Read the model definition and answer for the solid it produces. Units are mm, in the model's axes. Round coordinates to 2 decimals unless told otherwise and drop trailing zeros. Order: outer loops, then holes, each group sorted by start corner. A loop starts at its lowest first (then second) coordinate and runs counter-clockwise, first axis right, second up.
from build123d import *

# Parameters (mm, degrees)
SCHIZZO1_R                   = 1.5
ESTRUSIONE_ESTRUSIONE1_DEPTH = 3


with BuildPart() as part:
    # Schizzo1 → Estrusione-Estrusione1 (new body)
    with BuildSketch(Plane.XY):
        with BuildLine():
            Line((22, 5), (0, 5))
            ThreePointArc((0, 5), (-5, 0), (0, -5))
            Line((0, -5), (22, -5))
            ThreePointArc((22, -5), (25.445859834, -3.622989098), (26.993725045, -0.250420003))
            Line((26.993725045, -0.250420003), (45.041832618, 3.254653548))
            Line((45.041832618, 3.254653548), (50.666477461, 1.165785339))
            ThreePointArc((50.666477461, 1.165785339), (51.293977461, 1.08172232), (51.921477461, 1.165785339))
            ThreePointArc((51.921477461, 1.165785339), (52.551477461, 1.081007878), (53.181477461, 1.165785339))
            ThreePointArc((53.181477461, 1.165785339), (53.811477461, 1.081063133), (54.441477461, 1.165785339))
            ThreePointArc((54.441477461, 1.165785339), (55.071477461, 1.081063133), (55.701477461, 1.165785339))
            Line((55.701477461, 1.165785339), (55.766477461, 1.165785339))
            ThreePointArc((55.766477461, 1.165785339), (60.745551277, 6.622757917), (54.856357382, 11.082255764))
            Line((54.856357382, 11.082255764), (22, 5))
        make_face()
        Circle(SCHIZZO1_R, mode=Mode.SUBTRACT)
        with Locations((22, 0)):
            Circle(SCHIZZO1_R, mode=Mode.SUBTRACT)
        with Locations((55.766477461, 6.165785339)):
            Circle(SCHIZZO1_R, mode=Mode.SUBTRACT)
    extrude(amount=ESTRUSIONE_ESTRUSIONE1_DEPTH)


solid = part.part
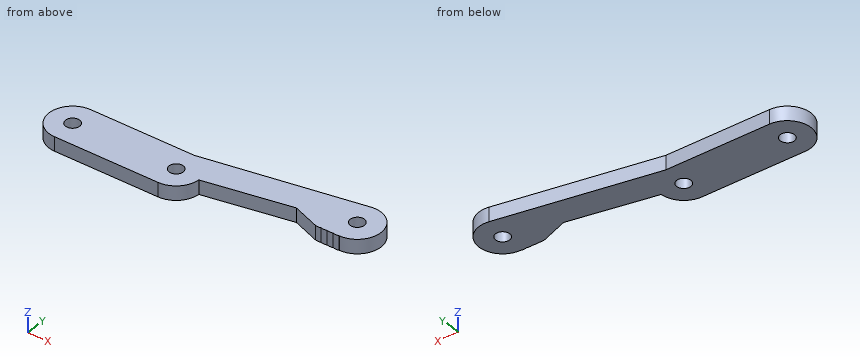
Q1. A cutting plane is placed at A-A, the plane z = 1.5. Give the vertices of the cut face in (x, y), plus the area to 3 significant figures.
Outcome:
outline: (0, -5) - (22, -5) arc R5 ccw to (26.99, -0.25) - (45.04, 3.25) - (50.67, 1.17) arc R2.38 ccw to (51.92, 1.17) arc R2.38 ccw to (53.18, 1.17) arc R2.38 ccw to (54.44, 1.17) arc R2.38 ccw to (55.7, 1.17) - (55.77, 1.17) arc R5 ccw (long way) to (54.86, 11.08) - (22, 5) - (0, 5) arc R5 ccw to start; hole circle Ø3 at (0, 0); hole circle Ø3 at (22, 0); hole circle Ø3 at (55.77, 6.17)
area: 526 mm2
Q2. A cutting plane is placed at B-B, the plane x = 18. Give the vertices of the cut face in (y, z).
Outcome:
outline: (-5, 0) - (5, 0) - (5, 3) - (-5, 3) - close
Q3. Flat-ended cylindrical pins translate along their axes: pin 1 (2.5 mm diameter, centred on x = 0, y = 0, fed in from +Z); pin 2 (1 mm diameter, centred on x = 30.5, z = 2, fed in from +Y); pin 3 (1 mm diameter, centred on x = 10.5, z = 1.5, fed in from +Y). Find the tip coordinate at first contact, or state that the pin passes through.
Outcome:
pin 1: passes through
pin 2: stops at y = 6.67
pin 3: stops at y = 5
Q4. A cutting plane is placed at C-C, the plane y = -3. Give the vertices of the cut face in (x, z), plus the area to 3 significant figures.
Outcome:
outline: (-4, 0) - (26, 0) - (26, 3) - (-4, 3) - close
area: 90.0 mm2
Q5. Straight lines are drawn through the part: probe 1 along Y at (x, z) = (22, 2.1); probe 2 along Y at (x, z) = (8, 2.3); probe 3 along Y at (x, z) = (-1, 1.25). For each, find the intervals that lie inside material, in ascending order.
Outcome:
probe 1: y = -5 to -1.5, 1.5 to 5
probe 2: y = -5 to 5
probe 3: y = -4.9 to -1.12, 1.12 to 4.9
